```python
from build123d import *

# Parameters (mm, degrees)
SKETCH_1_W          = 45
SKETCH_1_H          = 10
SKETCH_1_R          = 1.6
EXTRUDE_1_DEPTH     = 5
FILLET_1_RADIUS     = 5
FILLET_1_LENGTH     = 10
FILLET_2_RADIUS     = 5
FILLET_2_LENGTH     = 10
EXTRUDE_2_DEPTH     = 25
FILLET_8_R          = 1
CUT_EXTRUDE_START   = -20
CUT_EXTRUDE_1_DEPTH = 10


with BuildPart() as part:
    # Эскиз1 → Бобышка-Вытянуть1 (new, symmetric)
    with BuildSketch(Plane.XY):
        Rectangle(SKETCH_1_W, SKETCH_1_H)
        with Locations((-15, 0)):
            Circle(SKETCH_1_R, mode=Mode.SUBTRACT)
        with Locations(Location((15, 0, 0), (0, 0, 180))):
            Circle(SKETCH_1_R, mode=Mode.SUBTRACT)
    extrude(amount=EXTRUDE_1_DEPTH, both=True)

    # Скругление1: full round fillet: the end face becomes a half cylinder, R = half its width
    fillet_1_face = Plane((-22.5, 0, 0), x_dir=(0, 0, 1), z_dir=(-1, 0, 0))  # on the end face: x along it, z out of the body
    fillet_1_slab = fillet_1_face.offset(-FILLET_1_RADIUS / 2) * Box(FILLET_1_LENGTH, 2 * FILLET_1_RADIUS, FILLET_1_RADIUS, mode=Mode.PRIVATE)  # the body's end, R deep
    fillet_1_round = Plane((-17.5, 0, 0), x_dir=(-1, 0, 0), z_dir=(0, 0, 1)) * Cylinder(FILLET_1_RADIUS, FILLET_1_LENGTH, mode=Mode.PRIVATE)  # its axis R under the face
    add(fillet_1_slab - fillet_1_round, mode=Mode.SUBTRACT)

    # Скругление2: full round fillet: the end face becomes a half cylinder, R = half its width
    fillet_2_face = Plane((22.5, 0, 0), x_dir=(0, 0, -1), z_dir=(1, 0, 0))  # on the end face: x along it, z out of the body
    fillet_2_slab = fillet_2_face.offset(-FILLET_2_RADIUS / 2) * Box(FILLET_2_LENGTH, 2 * FILLET_2_RADIUS, FILLET_2_RADIUS, mode=Mode.PRIVATE)  # the body's end, R deep
    fillet_2_round = Plane((17.5, 0, 0), x_dir=(1, 0, 0), z_dir=(0, 0, -1)) * Cylinder(FILLET_2_RADIUS, FILLET_2_LENGTH, mode=Mode.PRIVATE)  # its axis R under the face
    add(fillet_2_slab - fillet_2_round, mode=Mode.SUBTRACT)

    # Эскиз2 → Бобышка-Вытянуть2 (add)
    with BuildSketch(Plane(origin=(0, 5, 0), x_dir=(1, 0, 0), z_dir=(0, 1, 0))):
        with BuildLine():
            Line((-6, 1.3), (6, 1.3))
            ThreePointArc((6, 1.3), (6.919238816, 0.919238816), (7.3, 0))
            Line((7.3, 0), (7.3, -0.2))
            ThreePointArc((7.3, -0.2), (7.349128161, -0.758575559), (7.49500416, -1.3))
            Line((7.49500416, -1.3), (-7.49500416, -1.3))
            ThreePointArc((-7.49500416, -1.3), (-7.349128161, -0.758575559), (-7.3, -0.2))
            Line((-7.3, -0.2), (-7.3, 0))
            ThreePointArc((-7.3, 0), (-6.919238816, 0.919238816), (-6, 1.3))
        make_face()
    extrude(amount=EXTRUDE_2_DEPTH)

    # Скругление8
    fillet_8_edges = [part.edges().sort_by_distance(p)[0] for p in [
        (0, 5, 1.3),
    ]]
    fillet(fillet_8_edges, radius=FILLET_8_R)
    fillet_8_2_edges = [part.edges().sort_by_distance(p)[0] for p in [
        (-7.349128161, 5, 0.758575559),
        (7.349128161, 5, 0.758575559),
        (7.3, 5, 0.1),
        (6.919238816, 5, -0.919238816),
        (0, 5, -1.3),
        (-6.919238816, 5, -0.919238816),
        (-7.3, 5, 0.1),
    ]]
    fillet(fillet_8_2_edges, radius=FILLET_8_R - 0.0001)  # a hair under: the kernel refuses the full size

    # Эскиз3 → Вырез-Вытянуть1 (cut)
    with BuildSketch(Plane(origin=(0, 30, 0), x_dir=(1, 0, 0), z_dir=(0, 1, 0)).offset(CUT_EXTRUDE_START)):
        with BuildLine():
            Line((6.3, -0.2), (6.3, 0))
            ThreePointArc((6.3, 0), (6.212132034, 0.212132034), (6, 0.3))
            Line((6, 0.3), (-6, 0.3))
            ThreePointArc((-6, 0.3), (-6.212132034, 0.212132034), (-6.3, 0))
            Line((-6.3, 0), (-6.3, -0.2))
            ThreePointArc((-6.3, -0.2), (-6.300297672, -0.250003544), (-6.301190645, -0.3))
            Line((-6.301190645, -0.3), (6.301190645, -0.3))
            ThreePointArc((6.301190645, -0.3), (6.300297672, -0.250003544), (6.3, -0.2))
        make_face()
    extrude(amount=-CUT_EXTRUDE_1_DEPTH, mode=Mode.SUBTRACT)


solid = part.part
```
Source: CAD feature listing. Evaluate the final solid. Frame: model axes, mm. A direction names the side the tool comes from. Give positions to 0.01 mm unless a question says otherwise; leave off trailing zeros. Write each loop counter-clockwise with the first axis right and the second up, starting at its lowest first coordinate (ties: lowest second). Pieces come first, ordered by that corner, then holes.
1. Section query A-A (x = -15). Return the cut outline in (y, z), then the cut area to 3 significant figures.
2. Section query D-D (y = 18.5). Return the cut outline in (x, z) (3 decimals).
3. Access query for faces 1 (the face through (-7.35, 17.83, 0.77)), 2 (the face through (0, 18, 1.3)), 3 (the face through (0, 5, -0.3)), 4 (the face through (0, 30, 0)), 5 (the face through (6.91, 17.83, -0.93)). Directions: +Z, -Z, +X, -X, +Y, -Y. A direction counts if a zero-diameter tool reaches every point of the face in a straight line with its end or side. Return the directions, or none.
4. First-contact query: pin 1 (7.5 mm diameter, centred on x = -1.5, y = 21.5, fed in from +Z); pin 2 (4 mm diameter, centred on y = 17, z = 2.5, fed in from -X) (3 decimals); pin 3 (3.5 mm diameter, centred on x = -1, y = 15.5, fed in from -Z). Flat tips, straight axial feed; report the tip coordinate or a pass-through.
5. Section query B-B (y = 4). Return the cut outline in (x, z).
6. Pull-direction query (Y, two-part tool) for faces 6 (the face through (22.5, 0.1, -0.1)), 7 (the face through (0, 5, 0.3)), 8 (the face through (0.084, 5.285, -1.601)); classes: +Y half, -Y half, draft (parallel to the pull), parting line (faces both ways), or undercut.
7. Section query C-C (x = -4). Return the cut outline in (y, z).
8. Material intervals for line 1 along Y through (x, z) = (-15, 0.25); line 2 along Z through (x, y) = (-0.5, 2.5); line 3 along Z through (x, y) = (2, 7), sorted ascending.
Output values:
1. outline: (-5, -5) - (-1.6, -5) - (-1.6, 5) - (-5, 5) - close; (1.6, -5) - (5, -5) - (5, 5) - (1.6, 5) - close
1. area: 68.0 mm2
2. outline: (-7.495, 1.3) arc R3.2 cw to (-7.3, 0.2) - (-7.3, 0) arc R1.3 ccw to (-6, -1.3) - (6, -1.3) arc R1.3 ccw to (7.3, 0) - (7.3, 0.2) arc R3.2 cw to (7.495, 1.3) - close
3. face 1: -Z, -X, +Y
3. face 2: +Z, +X, -X, +Y
3. face 3: none
3. face 4: +Z, -Z, +X, -X, +Y
3. face 5: -Z, +X, +Y
4. pin 1: stops at z = 1.3
4. pin 2: stops at x = -7.495
4. pin 3: stops at z = -1.3
5. outline: (-20.5, -5) - (20.5, -5) - (20.5, 5) - (-20.5, 5) - close; hole (-6.3, 0) arc R0.3 ccw to (-6, -0.3) - (6, -0.3) arc R0.3 ccw to (6.3, 0) - (6.3, 0.2) arc R4.2 cw to (6.3, 0.3) - (-6.3, 0.3) arc R4.2 cw to (-6.3, 0.2) - close
6. face 6: parting line
6. face 7: undercut
6. face 8: +Y half
7. outline: (-5, -5) - (5, -5) - (5, -2.3) arc R1 cw to (6, -1.3) - (30, -1.3) - (30, 1.3) - (6, 1.3) arc R1 cw to (5, 2.3) - (5, 5) - (-5, 5) - close; hole (0, -0.3) - (10, -0.3) - (10, 0.3) - (0, 0.3) - close
8. line 1: y = -5 to -1.6, 1.6 to 5
8. line 2: z = -5 to -0.3, 0.3 to 5
8. line 3: z = -1.3 to -0.3, 0.3 to 1.3
